Autodesk Inventor part; units mm, degrees
ref_plane "YZ Plane" through (0, 0, 0) normal (1, 0, 0) x (0, 1, 0)
ref_plane "XZ Plane" through (0, 0, 0) normal (0, 1, 0) x (-1, 0, 0)
ref_plane "XY Plane" through (0, 0, 0) normal (0, 0, 1) x (1, 0, 0)
sketch "Sketch1" plane through (0, 0, 0) normal (0, 1, 0) x (-1, 0, 0)
  line L0 (5.8164, 600.598) -> (-19.5836, 600.598)
  line L1 (-19.5836, 600.598) -> (-19.5836, -21.702)
  line L2 (-19.5836, -21.702) -> (5.8164, -21.702)
  line L3 (5.8164, -21.702) -> (5.8164, 600.598)
  point P0 (0, 0)
  dimension "d0" = 25.4
  dimension "d1" = 622.3
extrude "Extrusion1" add sketch "Sketch1" along normal blind 50.8
shell "Shell1" thickness 3.175 removed faces 2 at (2.6503, 33.8667, 600.598) at (11.117, 33.8667, -21.702)
sketch "Sketch2" plane through (0, 50.8, 0) normal (0, 1, 0) x (1, 0, 0)
  circle A0 centre (6.8836, -587.898) radius 2.5019
  line L0 (-5.8164, -600.598) -> (19.5836, -600.598)
  circle A1 centre (6.8836, -575.198) radius 2.5019
  circle A2 centre (6.8836, -562.498) radius 2.5019
  circle A3 centre (6.8836, 9.002) radius 2.5019
  circle A4 centre (6.8836, -3.698) radius 2.5019
  circle A5 centre (6.8836, -16.398) radius 2.5019
  line L1 (19.5836, 21.702) -> (-5.8164, 21.702)
  point P0 (0, 0)
  dimension "d5" = 5.0038
  dimension "d6" = 12.7
  dimension "d7" = 5.0038
  dimension "d8" = 5.0038
  dimension "d9" = 12.7
  dimension "d10" = 12.7
  dimension "d11" = 5.0038
  dimension "d12" = 5.0038
  dimension "d13" = 5.0038
  dimension "d14" = 12.7
  dimension "d15" = 12.7
  dimension "d16" = 12.7
extrude "Extrusion2" cut sketch "Sketch2" against normal blind 50.8
sketch "Sketch3" plane through (19.5836, 0, 600.598) normal (1, 0, 0) x (0, 0, -1)
  line L0 (0, 0) -> (0, 50.8) construction
  line L1 (622.3, 0) -> (622.3, 50.8) construction
  circle A0 centre (222.25, 25.4) radius 14.2875
  circle A1 centre (400.05, 25.4) radius 14.2875
  point P0 (600.598, 0)
  dimension "d21" = 28.575
  dimension "d22" = 28.575
hole "Hole1" at (19.5836, 25.4, 378.348) at (19.5836, 25.4, 200.548) direction (-1, 0, 0) diameter 28.575 end through all
sketch "Sketch4" plane through (0, 50.8, 0) normal (0, 1, 0) x (1, 0, 0)
  circle A0 centre (6.8836, -378.348) radius 3.175
  line L0 (-5.8164, -600.598) -> (19.5836, -600.598)
  circle A1 centre (6.8836, -200.548) radius 3.175
  line L1 (19.5836, 21.702) -> (-5.8164, 21.702)
  point P0 (0, 0)
  point P1 (6.8836, -600.598)
  dimension "d30" = 6.35
  dimension "d31" = 222.25
  dimension "d32" = 6.35
  dimension "d33" = 222.25
hole "Hole2" at (6.8836, 50.8, 378.348) at (6.8836, 50.8, 200.548) direction (0, -1, 0) diameter 6.35 end through all
properties part number "middle_alum_swerve" material "Aluminum 6061"
Work out the finished part from the listing and answer in its coordinate system (mm). A direction names the side the tool comes from. Coordinates: 2 decimals unless noted, no trailing zeros. Order: outer loops, then holes, each group sorted by start corner. A loop starts at its lowest first (then second) coordinate and runs counter-clockwise, first axis right, second up. Notation, with made-up numbers: (-16, 51.5) - (-4, 51.5) arc R23 ccw to (-4, 83.5) - close; hole circle Ø10 at (-29, 33.5). An arc over 180 degrees is marked (long way). Answer as a JSON object with one key per item and string values.
1. The mould has two halves that part along X. Classify faces 1 (the face through (-4.25, 21.11, 186.92)), 2 (the face through (-5.816, 25, 285)), 3 (the face through (19.584, 25, 294)), 4 (the face through (16.409, 25, 294)): +X half, -X half, draft (parallel to the pull), parting line (faces both ways), or undercut.
Output values:
{"face 1": "draft", "face 2": "-X half", "face 3": "+X half", "face 4": "undercut"}
2. Find section B-B on z = 403. Determine the outline of the cut face in (x, y) (3 decimals).
Output values:
{"outline": "(-5.816, 0) - (19.584, 0) - (19.584, 50.8) - (-5.816, 50.8) - close; hole (-2.641, 3.175) - (16.409, 3.175) - (16.409, 47.625) - (-2.641, 47.625) - close"}
3. This flat-tipped pin is pushed along its axis until it touches: P1, Ø5.5, axis at x = 6.88, z = 200.55, coming from the -Y side. Where does it stop, or does it pass through?
Output values:
{"P1": "passes through"}
4. Find section A-A on y = 25.4. Determine the outline of the cut face in (x, z).
Output values:
{"outline": "(-5.82, -21.7) - (-2.64, -21.7) - (-2.64, 186.26) - (-5.82, 186.26) - close; (-5.82, 214.84) - (-2.64, 214.84) - (-2.64, 364.06) - (-5.82, 364.06) - close; (-5.82, 392.64) - (-2.64, 392.64) - (-2.64, 600.6) - (-5.82, 600.6) - close; (16.41, -21.7) - (19.58, -21.7) - (19.58, 186.26) - (16.41, 186.26) - close; (16.41, 214.84) - (19.58, 214.84) - (19.58, 364.06) - (16.41, 364.06) - close; (16.41, 392.64) - (19.58, 392.64) - (19.58, 600.6) - (16.41, 600.6) - close"}
5. A tool of negligible diameter and unlimited length cuts with its end or side. For faces 5 (the face through (17.97, 21.11, 364.72)), 6 (the face through (7, 47.625, 294)), from which of +Z, -Z, +X, -X, +Y, -Y can it reach the whole face along a straight path? Write none if from no direction.
Output values:
{"face 5": "+X, -X", "face 6": "+Z, -Z"}
6. Consider line 1 (Z direction, x = -4.2, y = 25.4); line 2 (Y direction, x = 15.25, z = 172) (3 decimals); line 3 (X direction, y = 34, z = 360.5). Determine where each line is inside the solid, lowest interval first.
Output values:
{"line 1": "z = -21.7 to 186.26, 214.84 to 364.06, 392.64 to 600.6", "line 2": "y = 0 to 3.175, 47.625 to 50.8", "line 3": "x = -5.82 to -2.64, 16.41 to 19.58"}
